Design review of the part shown in the three views and the two pictorial views. Dimensions are in mm from the part's minimum x, y and z. Coordinates: 2 decimals unless noted, no trailing zeros. Loops run counter-clockwise (first coordinate to the right, second up) from the corner with the lowest first, then second, coordinate; pieces in that order, holes last. Notation, with made-up numbers: M 49.25,-39 L 105.25,-39 A25 ccw 105.25,-13 Z; hole C -27,0 d10. An arc over 180 degrees is marked long. Use one line per item in the form item = value.
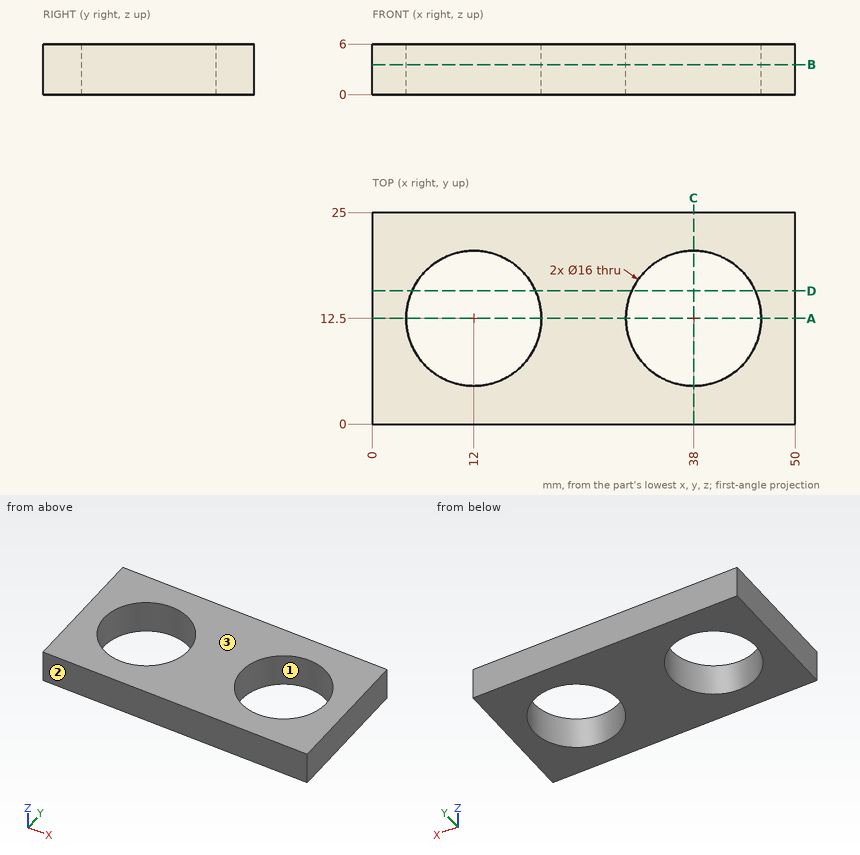
1. Add section D-D (y = 15.75). State the section outline as (x, z) points.
Response values:
outline = M 0,0 L 4.69,0 L 4.69,6 L 0,6 Z; M 19.31,0 L 30.69,0 L 30.69,6 L 19.31,6 Z; M 45.31,0 L 50,0 L 50,6 L 45.31,6 Z
2. Add section A-A (y = 12.5). State the section outline as (x, z) points, then the cut area to 3 significant figures.
Response values:
outline = M 0,0 L 4,0 L 4,6 L 0,6 Z; M 20,0 L 30,0 L 30,6 L 20,6 Z; M 46,0 L 50,0 L 50,6 L 46,6 Z
area = 108 mm^2
3. The part is to be moulded in two halves that separate along Y. For the marked faces 1, 2 and 3, say which applies: pulls with the +Y half, pulls with the -Y half, needs draft (parallel to the pull), parting line crosses it, or undercut.
Response values:
face_1 = undercut
face_2 = pulls with the -Y half
face_3 = needs draft
4. Add section C-C (x = 38). State the section outline as (y, z) points.
Response values:
outline = M 0,0 L 4.5,0 L 4.5,6 L 0,6 Z; M 20.5,0 L 25,0 L 25,6 L 20.5,6 Z
5. Wall thickness on line 1 along X through (y, z) = (12.5, 4); line 2 along Y through (x, z) = (12, 2.5); line 3 along X through (y, z) = (8, 5.4): over which ranges is each line inside the solid? List them lowest first. Write a range as from..to.
Response values:
line_1 = 0..4, 20..30, 46..50
line_2 = 0..4.5, 20.5..25
line_3 = 0..5.39, 18.61..31.39, 44.61..50
6. Add section B-B (z = 3.55). State the section outline as (x, y) points.
Response values:
outline = M 0,0 L 50,0 L 50,25 L 0,25 Z; hole C 12,12.5 d16; hole C 38,12.5 d16
